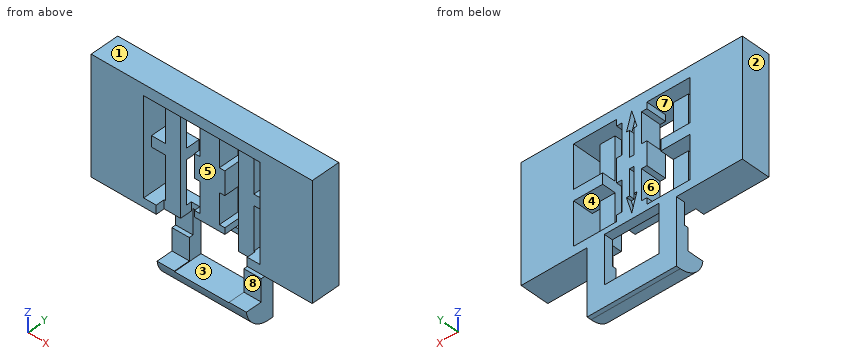
```python
from build123d import *

# Parameters (mm, degrees)
SKETCH1_W               = 64.75
SKETCH1_H               = 84.325
SKETCH1_R               = 1.35
BOSS_EXTRUDE1_DEPTH     = 25.4
CUT_EXTRUDE1_DEPTH      = 65.75
SKETCH5_W               = 58.925
SKETCH5_H               = 20.6375
CUT_EXTRUDE3_DEPTH      = 65.75
BOSS_EXTRUDE2_START     = 4.7625
SKETCH1_3_W             = 6.75
SKETCH1_3_H             = 6.75
SKETCH1_3_R             = 1.35
SKETCH1_3_H_2           = 3.175
BOSS_EXTRUDE2_DEPTH     = 6.35
SKETCH7_W               = 26.65
SKETCH7_H               = 58.925
CUT_EXTRUDE6_DEPTH      = 13.7
CUT_EXTRUDE6_DEPTH_BACK = 13.7
SKETCH8_W               = 64.75
SKETCH8_H               = 34.036
SKETCH8_W_2             = 4.064
SKETCH8_H_2             = 12.573
BOSS_EXTRUDE3_DEPTH     = 8.5
CUT_EXTRUDE7_START      = -8.5
SKETCH8_3_W             = 4.445
SKETCH8_3_H             = 12.573
CUT_EXTRUDE7_DEPTH      = 4
SKETCH8_4_W             = 4.445
SKETCH8_4_H             = 12.573
CUT_EXTRUDE8_DEPTH      = 2.54
SKETCH9_W               = 26.65
SKETCH9_H               = 86.865
SKETCH9_W_2             = 8.509
SKETCH9_H_2             = 3.175
CUT_EXTRUDE9_DEPTH      = 2.54
CUT_EXTRUDE10_DEPTH     = 1.5
SKETCH11_W              = 64.75
SKETCH11_H              = 84.325
CUT_EXTRUDE11_DEPTH     = 26.4
BOSS_EXTRUDE4_DEPTH     = 64.75
SKETCH15_W              = 19.304
SKETCH15_H              = 19.177
SKETCH15_W_2            = 16
SKETCH15_H_2            = 13.97
CUT_EXTRUDE12_DEPTH     = 9.5
SKETCH17_W              = 17.018
SKETCH17_H              = 2.54
CUT_EXTRUDE13_DEPTH     = 5.96


with BuildPart() as part:
    # Sketch1 → Boss-Extrude1 (new body)
    with BuildSketch(Plane(origin=(0, 0, 0), x_dir=(1, 0, 0), z_dir=(0, 1, 0))):
        Rectangle(SKETCH1_W, SKETCH1_H)
        with Locations((-29, 10.2125)):
            Circle(SKETCH1_R, mode=Mode.SUBTRACT)
        with Locations((-29, -38.7875)):
            Circle(SKETCH1_R, mode=Mode.SUBTRACT)
        with Locations((29, 10.2125)):
            Circle(SKETCH1_R, mode=Mode.SUBTRACT)
        with Locations((29, -38.7875)):
            Circle(SKETCH1_R, mode=Mode.SUBTRACT)
    extrude(amount=BOSS_EXTRUDE1_DEPTH)

    # Sketch3 → Cut-Extrude1 (cut, through all)
    with BuildSketch(Plane(origin=(32.375, 0, 0), x_dir=(0, 0, -1), z_dir=(1, 0, 0))):
        Polygon((42.1625, 18.034), (23.1125, 18.669), (23.1125, 12.7), (42.1625, 12.7), align=None)
    extrude(amount=-CUT_EXTRUDE1_DEPTH, mode=Mode.SUBTRACT)

    # Sketch5 → Cut-Extrude3 (cut, through all)
    with BuildSketch(Plane(origin=(32.375, 0, 0), x_dir=(0, 0, -1), z_dir=(1, 0, 0))):
        with Locations((-12.7, 15.08125)):
            Rectangle(SKETCH5_W, SKETCH5_H)
    extrude(amount=-CUT_EXTRUDE3_DEPTH, mode=Mode.SUBTRACT)

    # Sketch1<3> → Boss-Extrude2 (add)
    with BuildSketch(Plane(origin=(0, 0, 0), x_dir=(1, 0, 0), z_dir=(0, 1, 0)).offset(BOSS_EXTRUDE2_START)):
        with Locations((29, -38.7875)):
            Rectangle(SKETCH1_3_W, SKETCH1_3_H)
        with Locations((29, -38.7875)):
            Circle(SKETCH1_3_R, mode=Mode.SUBTRACT)
        with Locations((-29, -38.7875)):
            Rectangle(SKETCH1_3_W, SKETCH1_3_H)
        with Locations((-29, -38.7875)):
            Circle(SKETCH1_3_R, mode=Mode.SUBTRACT)
        with Locations((-29, 10.2125)):
            Rectangle(SKETCH1_3_W, SKETCH1_3_H)
        with Locations((-29, 10.2125)):
            Circle(SKETCH1_3_R, mode=Mode.SUBTRACT)
        with Locations((29, 10.2125)):
            Rectangle(SKETCH1_3_W, SKETCH1_3_H)
        with Locations((29, 10.2125)):
            Circle(SKETCH1_3_R, mode=Mode.SUBTRACT)
        with Locations((-29, 15.175)):
            Rectangle(SKETCH1_3_W, SKETCH1_3_H_2)
        with Locations((29, 15.175)):
            Rectangle(SKETCH1_3_W, SKETCH1_3_H_2)
    extrude(amount=BOSS_EXTRUDE2_DEPTH)

    # Sketch7 → Cut-Extrude6 (cut, two sides)
    with BuildSketch(Plane(origin=(0, 12.7, 0), x_dir=(1, 0, 0), z_dir=(0, 1, 0))) as cut_extrude6_sk:
        Rectangle(SKETCH7_W, SKETCH7_H)
    extrude(amount=CUT_EXTRUDE6_DEPTH, mode=Mode.SUBTRACT)
    extrude(cut_extrude6_sk.sketch, amount=-CUT_EXTRUDE6_DEPTH_BACK, mode=Mode.SUBTRACT)

    # Sketch8 → Boss-Extrude3 (add)
    with BuildSketch(Plane.XZ):
        with Locations((0, 59.1805)):
            Rectangle(SKETCH8_W, SKETCH8_H)
        with Locations((-14.986, 50.989)):
            Rectangle(SKETCH8_W_2, SKETCH8_H_2, mode=Mode.SUBTRACT)
        with Locations((-14.986, 66.737)):
            Rectangle(SKETCH8_W_2, SKETCH8_H_2, mode=Mode.SUBTRACT)
        Polygon((-8.509, 73.0235), (-4.445, 73.0235), (-4.445, 71.182), (-2.8575, 71.182), (-2.8575, 62.292), (-4.445, 62.292), (-4.445, 55.434), (-2.8575, 55.434), (-2.8575, 46.544), (-4.445, 46.544), (-4.445, 44.7025), (-8.509, 44.7025), align=None, mode=Mode.SUBTRACT)
        Polygon((4.445, 73.0235), (8.509, 73.0235), (8.509, 44.7025), (4.445, 44.7025), (4.445, 46.544), (2.8575, 46.544), (2.8575, 55.434), (4.445, 55.434), (4.445, 62.292), (2.8575, 62.292), (2.8575, 71.182), (4.445, 71.182), align=None, mode=Mode.SUBTRACT)
        with Locations((14.986, 66.737)):
            Rectangle(SKETCH8_W_2, SKETCH8_H_2, mode=Mode.SUBTRACT)
        with Locations((14.986, 50.989)):
            Rectangle(SKETCH8_W_2, SKETCH8_H_2, mode=Mode.SUBTRACT)
    extrude(amount=-BOSS_EXTRUDE3_DEPTH)

    # Sketch8<3> → Cut-Extrude7 (cut)
    with BuildSketch(Plane.XZ.offset(CUT_EXTRUDE7_START)):
        with Locations((-10.7315, 50.989)):
            Rectangle(SKETCH8_3_W, SKETCH8_3_H)
        with Locations((10.7315, 50.989)):
            Rectangle(SKETCH8_3_W, SKETCH8_3_H)
        with Locations((-10.7315, 66.737)):
            Rectangle(SKETCH8_3_W, SKETCH8_3_H)
        with Locations((10.7315, 66.737)):
            Rectangle(SKETCH8_3_W, SKETCH8_3_H)
    extrude(amount=CUT_EXTRUDE7_DEPTH, mode=Mode.SUBTRACT)

    # Sketch8<4> → Cut-Extrude8 (cut)
    with BuildSketch(Plane.XZ):
        with Locations((10.7315, 50.989)):
            Rectangle(SKETCH8_4_W, SKETCH8_4_H)
        with Locations((-10.7315, 50.989)):
            Rectangle(SKETCH8_4_W, SKETCH8_4_H)
        with Locations((10.7315, 66.737)):
            Rectangle(SKETCH8_4_W, SKETCH8_4_H)
        with Locations((-10.7315, 66.737)):
            Rectangle(SKETCH8_4_W, SKETCH8_4_H)
        Polygon((-4.445, 46.544), (-4.445, 44.7025), (4.445, 44.7025), (4.445, 46.544), (2.8575, 46.544), (2.8575, 49.084), (2.8575, 52.894), (2.8575, 55.434), (4.445, 55.434), (4.445, 57.2755), (4.445, 60.4505), (4.445, 62.292), (2.8575, 62.292), (2.8575, 64.832), (2.8575, 68.642), (2.8575, 71.182), (4.445, 71.182), (4.445, 73.0235), (-4.445, 73.0235), (-4.445, 71.182), (-2.8575, 71.182), (-2.8575, 68.642), (-2.8575, 64.832), (-2.8575, 62.292), (-4.445, 62.292), (-4.445, 60.4505), (-4.445, 57.2755), (-4.445, 55.434), (-2.8575, 55.434), (-2.8575, 52.894), (-2.8575, 49.084), (-2.8575, 46.544), align=None)
    extrude(amount=-CUT_EXTRUDE8_DEPTH, mode=Mode.SUBTRACT)

    # Sketch9 → Cut-Extrude9 (cut)
    with BuildSketch(Plane.XZ):
        with Locations((0, 1.27)):
            Rectangle(SKETCH9_W, SKETCH9_H)
        with Locations((-12.7635, 58.863)):
            Rectangle(SKETCH9_W_2, SKETCH9_H_2)
        with Locations((12.7635, 58.863)):
            Rectangle(SKETCH9_W_2, SKETCH9_H_2)
    extrude(amount=-CUT_EXTRUDE9_DEPTH, mode=Mode.SUBTRACT)

    # Sketch10 → Cut-Extrude10 (cut)
    with BuildSketch(Plane(origin=(0, 8.5, 0), x_dir=(1, 0, 0), z_dir=(0, 1, 0))):
        Polygon((-0.635, -57.2755), (0.635, -57.2755), (0.635, -49.7825), (1.524, -49.7825), (0, -44.7025), (-1.524, -49.7825), (-0.635, -49.7825), align=None)
        Polygon((-0.635, -67.9435), (-0.635, -60.4505), (0.635, -60.4505), (0.635, -67.9435), (1.524, -67.9435), (0, -73.0235), (-1.524, -67.9435), align=None)
    extrude(amount=-CUT_EXTRUDE10_DEPTH, mode=Mode.SUBTRACT)

    # Sketch11 → Cut-Extrude11 (cut, through all)
    with BuildSketch(Plane.XZ):
        Rectangle(SKETCH11_W, SKETCH11_H)
    extrude(amount=-CUT_EXTRUDE11_DEPTH, mode=Mode.SUBTRACT)

    # Sketch14 → Boss-Extrude4 (add)
    with BuildSketch(Plane(origin=(32.375, 0, 0), x_dir=(0, 0, -1), z_dir=(1, 0, 0))):
        with BuildLine():
            Line((-22.9855, 8.5), (-42.1625, 8.5))
            Line((-42.1625, 8.5), (-42.1625, 5.96))
            Line((-42.1625, 5.96), (-35.8125, 5.96))
            Line((-35.8125, 5.96), (-35.8125, 4.7625))
            Line((-35.8125, 4.7625), (-29.3355, 4.7625))
            Line((-29.3355, 4.7625), (-29.3355, 0))
            ThreePointArc((-29.3355, 0), (-24.798384872, 2.418674819), (-22.9855, 7.23))
            Line((-22.9855, 7.23), (-22.9855, 8.5))
        make_face()
    extrude(amount=-BOSS_EXTRUDE4_DEPTH)

    # Sketch15 → Cut-Extrude12 (cut, through all)
    with BuildSketch(Plane(origin=(0, 8.5, 0), x_dir=(1, 0, 0), z_dir=(0, 1, 0))):
        with Locations((-22.723, -32.574)):
            Rectangle(SKETCH15_W, SKETCH15_H)
        with Locations((0, -36.13)):
            Rectangle(SKETCH15_W_2, SKETCH15_H_2)
        with Locations((22.723, -32.574)):
            Rectangle(SKETCH15_W, SKETCH15_H)
    extrude(amount=-CUT_EXTRUDE12_DEPTH, mode=Mode.SUBTRACT)

    # Sketch17 → Cut-Extrude13 (cut)
    with BuildSketch(Plane.XZ):
        with Locations((0, 43.4325)):
            Rectangle(SKETCH17_W, SKETCH17_H)
    extrude(amount=-CUT_EXTRUDE13_DEPTH, mode=Mode.SUBTRACT)


solid = part.part
```
The listing builds one solid part. Answer for the finished solid, in the listing's coordinates (mm). Face numbers are marked on the shaded views. A direction names the side the tool comes from. Round coordinates to 2 decimals unless told otherwise and drop trailing zeros. Write each loop counter-clockwise with the first axis right and the second up, starting at its lowest first coordinate (ties: lowest second). Pieces come first, ordered by that corner, then holes. Notation, with made-up numbers: (-23, 18.5) -> (-6, 18.5) arc R13 ccw to (-6, 42.5) -> close; hole circle Ø8 at (-8.5, -11.5). An arc over 180 degrees is marked (long way). Write item = value, one per line.
1) Section B-B on x = -10 is taken. Write down the section's boundary in (y, z).
Check values:
outline = (0, 29.34) arc R7.29 ccw to (7.23, 22.99) -> (8.5, 22.99) -> (8.5, 44.7) -> (4.5, 44.7) -> (4.5, 57.28) -> (8.5, 57.28) -> (8.5, 60.45) -> (4.5, 60.45) -> (4.5, 73.02) -> (8.5, 73.02) -> (8.5, 76.2) -> (0, 76.2) -> (0, 73.02) -> (2.54, 73.02) -> (2.54, 42.16) -> (5.96, 42.16) -> (5.96, 35.81) -> (4.76, 35.81) -> (4.76, 29.34) -> close
2) For a pull along X with two mould halves and no side action, classify the marked faces 1, 2 and 3 as released by +X, released by -X, zero draft, split by the parting line, or undercut.
Check values:
face_1 = zero draft
face_2 = released by -X
face_3 = undercut
3) Straight lines are drawn through the part: line 1 along X through (y, z) = (5.5, 66.5) (1 decimal); line 2 along Z through (x, y) = (-16.5, 6.25); line 3 along X through (y, z) = (6.5, 61.5) (3 decimals). For each, find the intervals that lie inside material, in ascending order. Write a range as [from, to].
Check values:
line_1 = [-32.4, -17], [-2.9, 2.9], [17, 32.4]
line_2 = [42.16, 44.7], [57.28, 60.45], [73.02, 76.2]
line_3 = [-32.375, -17.018], [-4.445, 4.445], [17.018, 32.375]
4) Section A-A on z = 34.5 is taken. Write down the section's boundary in (x, y).
Check values:
outline = (-13.07, 4.76) -> (-8, 4.76) -> (-8, 8.5) -> (-13.07, 8.5) -> close; (8, 4.76) -> (13.07, 4.76) -> (13.07, 8.5) -> (8, 8.5) -> close
5) Which of the six approach directions +Z, -Z, +X, -X, +Y, -Y give full straight-line access (tool end or side, diameter ignored) to the marked faces 4, 5, 6, 7 and 8?
Check values:
face_4 = +Y
face_5 = -Y
face_6 = +Y, -Y
face_7 = none
face_8 = +X, -X, -Y
6) Section C-C on z = 52.5 is taken. Write down the section's boundary in (x, y) (1 decimal).
Check values:
outline = (-32.4, 0) -> (-17, 0) -> (-17, 8.5) -> (-32.4, 8.5) -> close; (-13, 2.5) -> (-8.5, 2.5) -> (-8.5, 4.5) -> (-13, 4.5) -> close; (-2.9, 2.5) -> (2.9, 2.5) -> (2.9, 8.5) -> (0.6, 8.5) -> (0.6, 7) -> (-0.6, 7) -> (-0.6, 8.5) -> (-2.9, 8.5) -> close; (8.5, 2.5) -> (13, 2.5) -> (13, 4.5) -> (8.5, 4.5) -> close; (17, 0) -> (32.4, 0) -> (32.4, 8.5) -> (17, 8.5) -> close
7) Given pin 1 (1.7 mm diameter, centred on x = 3.5, y = 4, fed in from -Z); pin 2 (4 mm diameter, centred on y = 4, z = 36, fed in from -X); pin 3 (4 mm diameter, centred on x = -14.5, y = 2.5, fed in from -Z), each flat-ended and moving along its own axis, determine where each tip first touches the part or whether it passes through.
Check values:
pin_1 = 23.38
pin_2 = -13.07
pin_3 = 23.79
